```python
from build123d import *

# Parameters (mm, degrees)
LINEAR_AUSTRAGEN_D_NN1_DEPTH      = 3
LINEAR_AUSTRAGEN_D_NN1_DEPTH_BACK = 3


with BuildPart() as part:
    # Skizze1 → Linear-Austragen-Dünn1 (new body, two sides)
    with BuildSketch(Plane(origin=(0, 0, 0), x_dir=(1, 0, 0), z_dir=(0, 1, 0))) as linear_austragen_d_nn1_sk:
        with BuildLine():
            Line((5.425321809, 4.783135297), (0.617779056, 5.339379556))
            ThreePointArc((0.617779056, 5.339379556), (-5.375, 0), (0.617779056, -5.339379556))
            Line((0.617779056, -5.339379556), (5.425321809, -4.783135297))
            ThreePointArc((5.425321809, -4.783135297), (6.11685444, -4.751365683), (6.806147081, -4.815415227))
            Line((6.806147081, -4.815415227), (67.493650964, -14.729735548))
            ThreePointArc((67.493650964, -14.729735548), (84.825, 0), (67.493650964, 14.729735548))
            Line((67.493650964, 14.729735548), (6.806147081, 4.815415227))
            ThreePointArc((6.806147081, 4.815415227), (6.11685444, 4.751365683), (5.425321809, 4.783135297))
        make_face()
        with BuildLine():
            Line((5.333373298, 3.988436945), (0.525830545, 4.544681203))
            ThreePointArc((0.525830545, 4.544681203), (-4.575, 0), (0.525830545, -4.544681203))
            Line((0.525830545, -4.544681203), (5.333373298, -3.988436945))
            ThreePointArc((5.333373298, -3.988436945), (6.135551151, -3.951584192), (6.935130614, -4.025881663))
            Line((6.935130614, -4.025881663), (67.622634497, -13.940201984))
            ThreePointArc((67.622634497, -13.940201984), (84.025, 0), (67.622634497, 13.940201984))
            Line((67.622634497, 13.940201984), (6.935130614, 4.025881663))
            ThreePointArc((6.935130614, 4.025881663), (6.135551151, 3.951584192), (5.333373298, 3.988436945))
        make_face(mode=Mode.SUBTRACT)
    extrude(amount=LINEAR_AUSTRAGEN_D_NN1_DEPTH)
    extrude(linear_austragen_d_nn1_sk.sketch, amount=-LINEAR_AUSTRAGEN_D_NN1_DEPTH_BACK)


solid = part.part
```
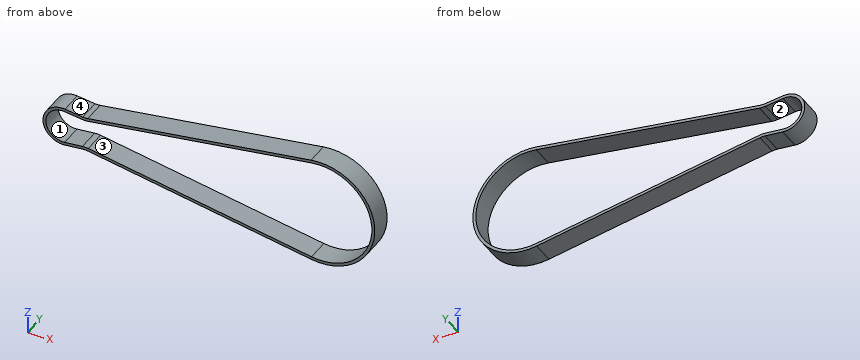
Work out the finished part from the listing and answer in its coordinate system (mm). Face numbers are marked on the shaded views. A direction names the side the tool comes from. Give positions to 0.01 mm unless a question says otherwise; leave off trailing zeros. Write each loop counter-clockwise with the first axis right and the second up, starting at its lowest first coordinate (ties: lowest second). Pieces come first, ordered by that corner, then holes.
(1) The part is cut by section A-A on x = 69.9. Write down the section's boundary in (y, z) (3 decimals).
Final values:
outline: (-3, -14.925) - (3, -14.925) - (3, -14.125) - (-3, -14.125) - close; (-3, 14.125) - (3, 14.125) - (3, 14.925) - (-3, 14.925) - close
(2) Straight lines are drawn through the part: line 1 (Z direction, x = 0, y = -0.7) (3 decimals); line 2 (X direction, y = 2.7, z = -2.5); line 3 (Z direction, x = 58, y = -1.9). For each, find the intervals that lie inside material, in ascending order.
Final values:
line 1: z = -5.375 to -4.575, 4.575 to 5.375
line 2: x = -4.76 to -3.83, 83.8 to 84.61
line 3: z = -13.18 to -12.37, 12.37 to 13.18
(3) Which of the six approach directions +Z, -Z, +X, -X, +Y, -Y give full straight-line access (tool end or side, diameter ignored) to the marked faces 3 and 4?
Final values:
face 3: +Y, -Y
face 4: +Z, +Y, -Y
(4) The part is cut by section B-B on z = 0. Write down the section's boundary in (x, y) (3 decimals), plus the area to 3 significant figures.
Final values:
outline: (-5.375, -3) - (-4.575, -3) - (-4.575, 3) - (-5.375, 3) - close; (84.025, -3) - (84.825, -3) - (84.825, 3) - (84.025, 3) - close
area: 9.60 mm2
(5) The mould has two halves that part along X. Classify the marked faces 1 and 2: pulls with the +X half, pulls with the -X half, needs draft (parallel to the pull), parting line crosses it, or undercut.
Final values:
face 1: undercut
face 2: undercut
(6) The part is cut by section C-C on y = -2.1. Write down the section's boundary in (x, z) (3 decimals).
Final values:
outline: (0.618, -5.339) - (5.425, -4.783) arc R5 cw to (6.806, -4.815) - (67.494, -14.73) arc R14.925 ccw (long way) to (67.494, 14.73) - (6.806, 4.815) arc R5 cw to (5.425, 4.783) - (0.618, 5.339) arc R5.375 ccw (long way) to start; hole (0.526, -4.545) - (5.333, -3.988) arc R5.8 cw to (6.935, -4.026) - (67.623, -13.94) arc R14.125 ccw (long way) to (67.623, 13.94) - (6.935, 4.026) arc R5.8 cw to (5.333, 3.988) - (0.526, 4.545) arc R4.575 ccw (long way) to start
(7) Flat-ended cylindrical pins translate along their axes: pin 1 Ø1 at (x, y) = (23, 1.5) entering from -Z; pin 2 Ø1.5 at (y, z) = (-1.5, 5.5) entering from +X. Find the tip coordinate at first contact, or state that the pin passes through.
Final values:
pin 1: stops at z = -7.54
pin 2: stops at x = 84.05
